Geometry: final body of the model. Coordinates: model frame, mm. Face numbers are marked on the shaded views. A direction names the side the tool comes from. Give positions to 0.01 mm unless a question says otherwise; leave off trailing zeros. Order: outer loops, then holes, each group sorted by start corner. A loop starts at its lowest first (then second) coordinate and runs counter-clockwise, first axis right, second up. Notation, with made-up numbers: (25.5, -12) - (78.5, -12) arc R19 ccw to (78.5, 14) - close; hole circle Ø4 at (15.5, 79). An arc over 180 degrees is marked (long way). Put each result on its own line as item: value. Start each with the question number.
1. Mould query, pull axis X, two halves, no side actions, for the marked faces 3, 4 and 5. Classes: pulls with the +X half, pulls with the -X half, needs draft (parallel to the pull), parting line crosses it, or undercut.
2. Set-up query: the marked faces 1 and 2. Return all of +Z, -Z, +X, -X, +Y, -Y with unobstructed straight access to the full face (end or side cutting, diameter ignored); none if empty.
3. Section A-A on y = 1. Return the cut outline in (x, z), plus the area to 3 significant figures.
4. Ray query, line 1 along Z through (x, y) = (0, -3.1); line 2 along Z through (x, y) = (0, -2); line 3 along Y through (x, z) = (6, 2). Return the intervals inside material, ascending. Write a range as from..to.
5. First-contact query: P1, Ø1.5, axis at x = 5.5, z = 6, coming from the -Y side; P2, Ø7, axis at x = 0, z = 0, coming from the -Y side; P3, Ø2, axis at y = 2, z = 5.5, coming from the -X side; P4, Ø4, axis at x = 6, y = -1.5, coming from the -Z side. Flat tips, straight axial feed; report the tip coordinate or a pass-through.
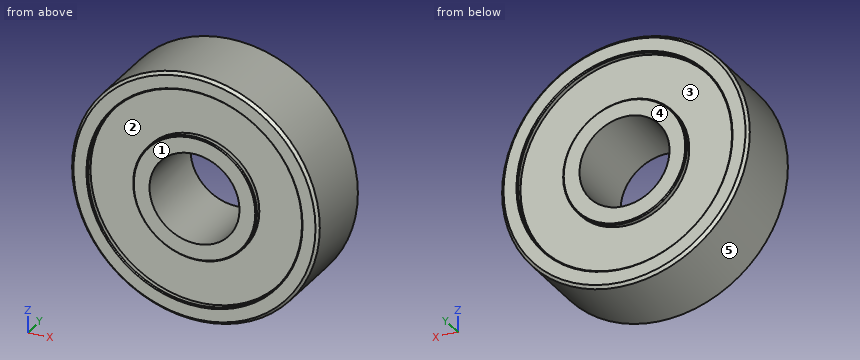
from build123d import *

# Parameters (mm, degrees)
F0_R     = 11
F0_R_2   = 4
F1_DEPTH = 3.5
F2_R     = 9.5
F2_R_2   = 5.5
F3_DEPTH = 0.5
F4_SIZE  = 0.25
F5_SIZE  = 0.1


# Not quite as in the source:
# - a pattern or mirror of a feature is missing from the dataset's text; its kind, count and spacing are read off the source's solid


with BuildPart() as f1:
    # F0 (on Front) → F1 (new body, symmetric)
    with BuildSketch(Plane.XZ):
        Circle(F0_R)
        Circle(F0_R_2, mode=Mode.SUBTRACT)
    extrude(amount=F1_DEPTH, both=True)

    # F2 (on face) → F3 (cut)
    with BuildSketch(Plane.XZ.offset(3.5)):
        Circle(F2_R)
        Circle(F2_R_2, mode=Mode.SUBTRACT)
    f3 = extrude(amount=-F3_DEPTH, mode=Mode.SUBTRACT)

    # F3_copies: F3 across plane
    add(f3.mirror(Plane.ZX), mode=Mode.SUBTRACT)

    # F4
    f4_edges = [f1.edges().sort_by_distance(p)[0] for p in [
        (-11, -3.5, 0),
        (-11, 3.5, 0),
    ]]
    chamfer(f4_edges, length=F4_SIZE)

    # F5
    f5_edges = [f1.edges().sort_by_distance(p)[0] for p in [
        (-9.5, -3.5, 0),
        (-5.5, -3.5, 0),
        (-9.5, 3.5, 0),
        (-5.5, 3.5, 0),
    ]]
    chamfer(f5_edges, length=F5_SIZE)


solid = f1.part
Resolved:
1. face 3: undercut
1. face 4: needs draft
1. face 5: parting line crosses it
2. face 1: +Z, -Z, +X, -X, -Y
2. face 2: -Y
3. outline: circle Ø22 at (0, 0); hole circle Ø8 at (0, 0)
3. area: 330 mm^2
4. line 1: -11..-9.5, -5.5..-4, 4..5.5, 9.5..11
4. line 2: -11..-4, 4..11
4. line 3: -3..3
5. P1: y = -3
5. P2: through
5. P3: x = -10.04
5. P4: z = -10.25
